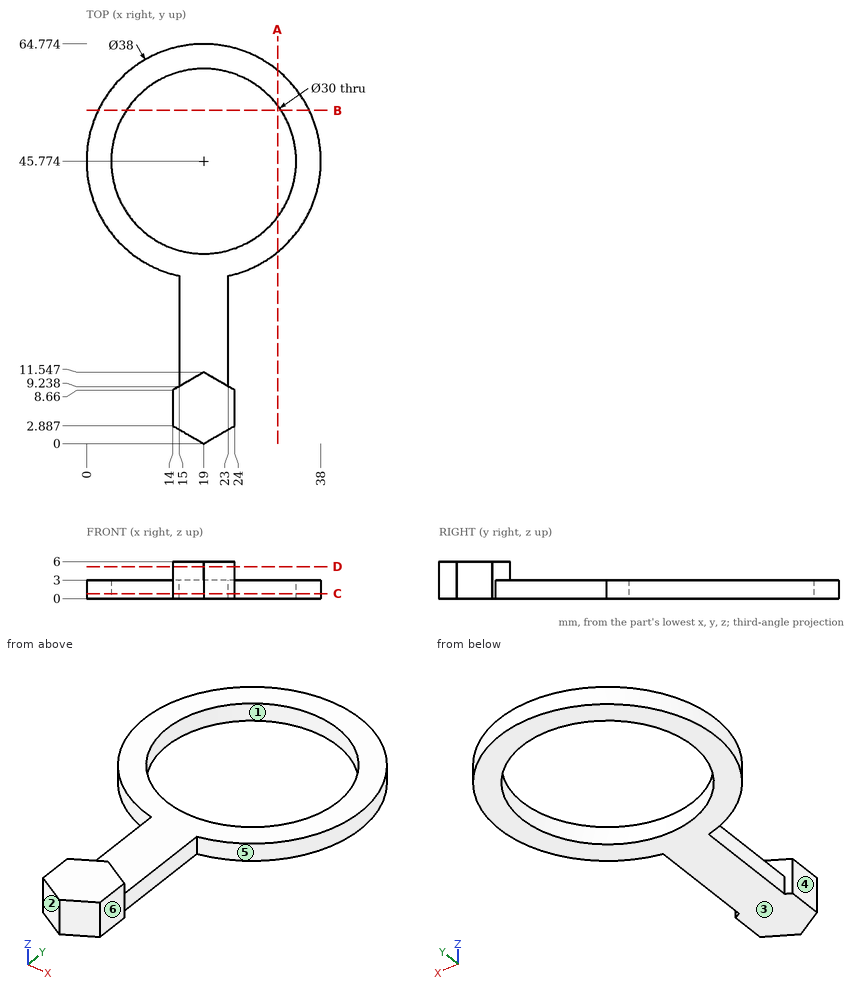
For this review, use the dimensioned drawing (mm, ordinates from the lowest corner) and the shaded views. A direction names the side the tool comes from. Round coordinates to 2 decimals unless told otherwise and drop trailing zeros. Write each loop counter-clockwise with the first axis right and the second up, starting at its lowest first coordinate (ties: lowest second). Pieces come first, ordered by that corner, then holes. Notation, with made-up numbers: (4.5, 38.25) -> (48.5, 38.25) arc R33 ccw to (48.5, 74.25) -> close; hole circle Ø4 at (-20.5, -7). An arc over 180 degrees is marked (long way). Answer in a Markdown table with one row per item.
Q1. For the marked faces 4, 5 and 6, list the 3-axis set-ups (+Z, -Z, +X, -X, +Y, -Y) from which the entire face can be reached by the end or side of a thin tool; tool diameter is ignored.
The answers:
| item | result |
|---|---|
| face 4 | +Z, -Z, -X, -Y |
| face 5 | +Z, -Z |
| face 6 | +Z, -Z, +X, -Y |
Q2. Draft analysis for pull direction Y (two halves, no side actions). For the marked faces 1, 2 and 3, state which applies: +Y half, -Y half, draft (parallel to the pull), parting line (faces both ways), or undercut.
The answers:
| item | result |
|---|---|
| face 1 | undercut |
| face 2 | -Y half |
| face 3 | draft |
Q3. Take a section at A-A, the plane x = 31. State the section outline as (y, z) points (1 decimal).
The answers:
| item | result |
|---|---|
| outline | (31, 0) -> (36.8, 0) -> (36.8, 3) -> (31, 3) -> close; (54.8, 0) -> (60.5, 0) -> (60.5, 3) -> (54.8, 3) -> close |
Q4. To check wall thickness, follow L1, parallel to Z at x = 32, y = 55; L2, parallel to X at y = 46, z = 1; L3, parallel to X at y = 11.5, z = 0.5. State the ranges of each line that lie inside material, in increasing order. Write a range as [from, to].
The answers:
| item | result |
|---|---|
| L1 | [0, 3] |
| L2 | [0, 4], [34, 38] |
| L3 | [15, 23] |
Q5. Take a section at D-D, the plane z = 5.2. State the section outline as (x, y) points.
The answers:
| item | result |
|---|---|
| outline | (14, 2.89) -> (19, 0) -> (24, 2.89) -> (24, 8.66) -> (19, 11.55) -> (14, 8.66) -> close |
Q6. Take a section at C-C, the plane z = 0.8. State the section outline as (x, y) points, then the cut area to 3 significant figures.
The answers:
| item | result |
|---|---|
| outline | (14, 2.89) -> (19, 0) -> (24, 2.89) -> (24, 8.66) -> (23, 9.24) -> (23, 27.2) arc R19 ccw (long way) to (15, 27.2) -> (15, 9.24) -> (14, 8.66) -> close; hole circle Ø30 at (19, 45.77) |
| area | 646 mm² |
Q7. Take a section at B-B, the plane y = 54. State the section outline as (x, z) points, then the cut area to 3 significant figures.
The answers:
| item | result |
|---|---|
| outline | (1.87, 0) -> (6.46, 0) -> (6.46, 3) -> (1.87, 3) -> close; (31.54, 0) -> (36.13, 0) -> (36.13, 3) -> (31.54, 3) -> close |
| area | 27.5 mm² |
Q8. Clearance check with flat-ended pins moving along their axes: pin 1 Ø3 at (y, z) = (15.5, 2) entering from -X; pin 2 Ø3 at (y, z) = (6.5, 2.5) entering from +X; pin 3 Ø4 at (x, y) = (13.5, 17) entering from +Z; pin 4 Ø1.5 at (y, z) = (46, 3.5) entering from +X. State where each tip first meets the part, or that it passes through.
The answers:
| item | result |
|---|---|
| pin 1 | x = 15 |
| pin 2 | x = 24 |
| pin 3 | z = 3 |
| pin 4 | x = 38 |
